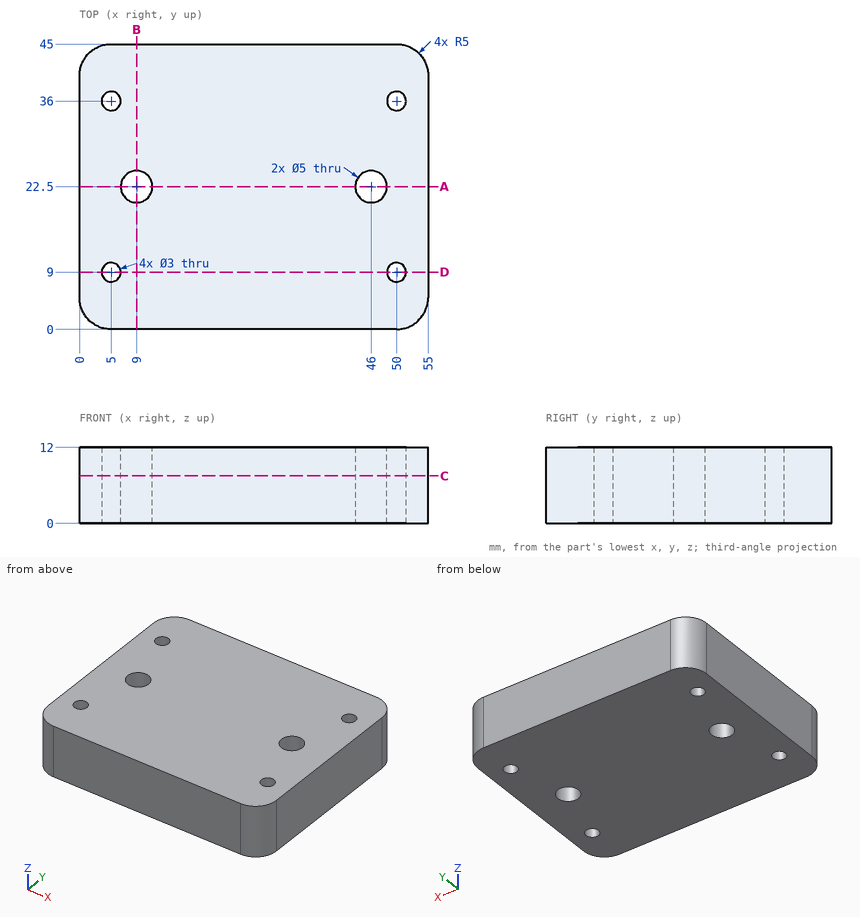
Here's the drawing with two shaded views (mm, measured from the low corner). I have some questions. Round coordinates to 2 decimals unless told otherwise and drop trailing zeros. Loops run counter-clockwise (first coordinate to the right, second up) from the corner with the lowest first, then second, coordinate; pieces in that order, holes last. Notation, with made-up numbers: M -12,21 L 43,21 A11 cw 43,34 Z; hole C 20,-11 d6. An arc over 180 degrees is marked long. Put each result on its own line as item: value.
Q1. Imagine slicing it at B-B (x = 9). Write out the boundary of the cut face in (y, z).
Check result:
outline: M 0,0 L 20,0 L 20,12 L 0,12 Z; M 25,0 L 45,0 L 45,12 L 25,12 Z
Q2. I need wall thicknesses on probe 1 along Y at (x, z) = (5, 8.75); probe 2 along Y at (x, z) = (46, 7.5); probe 3 along X at (y, z) = (8, 5.75). Which ranges of each line are inside material? Lowest first, please.
Check result:
probe 1: 0 to 7.5, 10.5 to 34.5, 37.5 to 45
probe 2: 0 to 20, 25 to 45
probe 3: 0 to 3.88, 6.12 to 48.88, 51.12 to 55
Q3. Imagine slicing it at D-D (y = 9). Write out the boundary of the cut face in (x, z).
Check result:
outline: M 0,0 L 3.5,0 L 3.5,12 L 0,12 Z; M 6.5,0 L 48.5,0 L 48.5,12 L 6.5,12 Z; M 51.5,0 L 55,0 L 55,12 L 51.5,12 Z
Q4. Imagine slicing it at C-C (z = 7.5). Write out the boundary of the cut face in (x, y).
Check result:
outline: M 0,5 A5 ccw 5,0 L 50,0 A5 ccw 55,5 L 55,40 A5 ccw 50,45 L 5,45 A5 ccw 0,40 Z; hole C 5,9 d3; hole C 5,36 d3; hole C 9,22.5 d5; hole C 46,22.5 d5; hole C 50,9 d3; hole C 50,36 d3
Q5. Imagine slicing it at A-A (y = 22.5). Write out the boundary of the cut face in (x, z).
Check result:
outline: M 0,0 L 6.5,0 L 6.5,12 L 0,12 Z; M 11.5,0 L 43.5,0 L 43.5,12 L 11.5,12 Z; M 48.5,0 L 55,0 L 55,12 L 48.5,12 Z
